from build123d import *

# Parameters (mm, degrees)
ESQUISSE1_R          = 1.65
ESQUISSE1_R_2        = 3.5
SHAPE_DEPTH          = 10
ESQUISSE6_W          = 10
ESQUISSE6_H          = 15
MAINSHAPE_DEPTH      = 30.25
ESQUISSE10_W         = 13.5
ESQUISSE10_H         = 12.85118471
SPACEREMOVER_DEPTH   = 13
ESQUISSE11_R         = 2.25
AXE_DEPTH            = 16
ESQUISSE12_R         = 3.7
BEARINGBOTTOM_DEPTH  = 3.2
BEARINGTOP_START     = -3.4
ESQUISSE14_R         = 3.7
BEARINGTOP_DEPTH     = 3.4
ESQUISSE15_R         = 2.25
AXEEND_DEPTH         = 1
ESQUISSE16_W         = 3
ESQUISSE16_H         = 7
AXELOCKER_DEPTH      = 10
ESQUISSE17_W         = 30.25
ESQUISSE17_H         = 0.85118471
RENFORCMENT_DEPTH    = 10
ESQUISSE18_W         = 30.25
ESQUISSE18_H         = 2
MASSREMOVER_DEPTH    = 10
CONG_1_R             = 4
ESQUISSE19_R         = 1
REMOVER_HELPER_DEPTH = 10


with BuildPart() as part:
    # Esquisse1 → Shape (new body)
    with BuildSketch(Plane.XY):
        with BuildLine():
            ThreePointArc((5, 10), (0, 15), (-5, 10))
            Line((-5, 10), (-5, -10))
            ThreePointArc((-5, -10), (0, -15), (5, -10))
            Line((5, -10), (5, 10))
        make_face()
        with Locations((0, 10)):
            Circle(ESQUISSE1_R, mode=Mode.SUBTRACT)
        Circle(ESQUISSE1_R_2, mode=Mode.SUBTRACT)
        with Locations((0, -10)):
            Circle(ESQUISSE1_R, mode=Mode.SUBTRACT)
    extrude(amount=SHAPE_DEPTH)

    # Esquisse6 → MainShape (add)
    with BuildSketch(Plane(origin=(5, 0, 0), x_dir=(0, 0, -1), z_dir=(1, 0, 0))):
        with Locations((-5, 0)):
            Rectangle(ESQUISSE6_W, ESQUISSE6_H)
    extrude(amount=MAINSHAPE_DEPTH)

    # Esquisse10 → SpaceRemover (cut)
    with BuildSketch(Plane(origin=(0, 0, 0), x_dir=(-1, 0, 0), z_dir=(0, 0, -1))):
        with Locations((-15.5, 1.074407645)):
            Rectangle(ESQUISSE10_W, ESQUISSE10_H)
    extrude(amount=-SPACEREMOVER_DEPTH, mode=Mode.SUBTRACT)

    # Esquisse11 → Axe (cut)
    with BuildSketch(Plane(origin=(35.25, 0, 0), x_dir=(0, 0, -1), z_dir=(1, 0, 0))):
        with Locations((-5, 0)):
            Circle(ESQUISSE11_R)
    extrude(amount=-AXE_DEPTH, mode=Mode.SUBTRACT)

    # Esquisse12 → BearingBottom (cut)
    with BuildSketch(Plane(origin=(8.75, 0, 0), x_dir=(0, 0, -1), z_dir=(1, 0, 0))):
        with Locations((-5, 0)):
            Circle(ESQUISSE12_R)
    extrude(amount=-BEARINGBOTTOM_DEPTH, mode=Mode.SUBTRACT)

    # Esquisse14 → BearingTop (cut)
    with BuildSketch(Plane.ZY.offset(-22.25).offset(BEARINGTOP_START)):
        with Locations(Location((5, 0, 0), (0, 0, 180))):
            Circle(ESQUISSE14_R)
    extrude(amount=BEARINGTOP_DEPTH, mode=Mode.SUBTRACT)

    # Esquisse15 → AxeEnd (cut)
    with BuildSketch(Plane(origin=(5.55, 0, 0), x_dir=(0, 0, -1), z_dir=(1, 0, 0))):
        with Locations((-5, 0)):
            Circle(ESQUISSE15_R)
    extrude(amount=-AXEEND_DEPTH, mode=Mode.SUBTRACT)

    # Esquisse16 → AxeLocker (cut)
    with BuildSketch(Plane(origin=(0, 0, 0), x_dir=(-1, 0, 0), z_dir=(0, 0, -1))):
        with Locations((-30.45, 0)):
            Rectangle(ESQUISSE16_W, ESQUISSE16_H)
    extrude(amount=-AXELOCKER_DEPTH, mode=Mode.SUBTRACT)

    # Esquisse17 → Renforcment (add)
    with BuildSketch(Plane(origin=(0, 0, 0), x_dir=(-1, 0, 0), z_dir=(0, 0, -1))):
        with Locations((-20.125, -7.925592355)):
            Rectangle(ESQUISSE17_W, ESQUISSE17_H)
    extrude(amount=-RENFORCMENT_DEPTH)

    # Esquisse18 → MassRemover (cut)
    with BuildSketch(Plane(origin=(0, 0, 0), x_dir=(-1, 0, 0), z_dir=(0, 0, -1))):
        with Locations((-20.125, 6.5)):
            Rectangle(ESQUISSE18_W, ESQUISSE18_H)
    extrude(amount=-MASSREMOVER_DEPTH, mode=Mode.SUBTRACT)

    # Congé1
    cong_1_edges = [part.edges().sort_by_distance(p)[0] for p in [
        (35.25, -8.35118471, 5),
        (5, -8.35118471, 5),
    ]]
    fillet(cong_1_edges, radius=CONG_1_R)

    # Esquisse19 → Remover helper (cut)
    with BuildSketch(Plane(origin=(4.55, 0, 0), x_dir=(0, 0, -1), z_dir=(1, 0, 0))):
        with Locations((-5, 0)):
            Circle(ESQUISSE19_R)
    extrude(amount=-REMOVER_HELPER_DEPTH, mode=Mode.SUBTRACT)


solid = part.part
Geometry: final body of the model. Coordinates: model frame, mm. A direction names the side the tool comes from. Give positions to 0.01 mm unless a question says otherwise; leave off trailing zeros. Order: outer loops, then holes, each group sorted by start corner. A loop starts at its lowest first (then second) coordinate and runs counter-clockwise, first axis right, second up. Notation, with made-up numbers: (56.5, -1.5) - (66.5, -1.5) arc R22 ccw to (66.5, 33.5) - close; hole circle Ø3 at (44.5, 54). An arc over 180 degrees is marked (long way). Use CSV: the item, a comma, the result in double quotes.
1. Section query A-A (x = 0). Output: boundary loops of the cut face in (y, z), plus the area to 3 significant figures.
Answers below:
outline,"(-15, 0) - (-11.65, 0) - (-11.65, 10) - (-15, 10) - close; (-8.35, 0) - (-3.5, 0) - (-3.5, 10) - (-8.35, 10) - close; (3.5, 0) - (8.35, 0) - (8.35, 10) - (3.5, 10) - close; (11.65, 0) - (15, 0) - (15, 10) - (11.65, 10) - close"
area,"164 mm2"
2. Access query for faces 5 (the face through (16, -5.351, 5)), 6 (the face through (23.97, -1.11, 1.47)), 7 (the face through (7, 5.5, 5)). Directions: +Z, -Z, +X, -X, +Y, -Y. A direction counts if a zero-diameter tool reaches every point of the face in a straight line with its end or side. Return the directions, or none.
Answers below:
face 5,"+Z, -Z, +Y"
face 6,"none"
face 7,"+Z, -Z, +X, +Y"
3. Section query C-C (z = 5). Give the number of separate pieces and of enclosed holes in the cut face, plus the area to 3 significant figures.
Answers below:
separate pieces,"3"
enclosed holes,"2"
area,"385 mm2"
4. Contact query for flat-ended pins moving along their axis: pin 1 (4 mm diameter, centred on x = 0, y = 10, fed in from -Z); pin 2 (4 mm diameter, centred on x = 0, y = 0, fed in from -Z); pin 3 (1 mm diameter, centred on x = 17.5, z = 3.5, fed in from +Y); pin 4 (2.5 mm diameter, centred on x = 30.5, z = 3.5, fed in from -Y). Output: stop coordinate, or through.
Answers below:
pin 1,"z = 0"
pin 2,"through"
pin 3,"y = -5.35"
pin 4,"y = -8.35"
5. Section query D-D (x = 26.5). Output: boundary loops of the cut face in (y, z).
Answers below:
outline,"(-8.35, 0) - (5.5, 0) - (5.5, 10) - (-8.35, 10) - close; hole circle Ø4.5 at (0, 5)"
6. Section query B-B (y = 5). Output: boundary loops of the cut face in (x, z), plus the area to 4 significant figures.
Answers below:
outline,"(-5, 0) - (8.75, 0) - (8.75, 10) - (-5, 10) - close; (22.25, 0) - (35.25, 0) - (35.25, 10) - (22.25, 10) - close"
area,"267.5 mm2"
7. Mould query, pull axis Y, two halves, no side actions, for faces 1 (the face through (8.75, 4, 4)), 2 (the face through (7.172, -1.417, 1.582)), 3 (the face through (4.55, 1, 4)), 4 (the face through (20, -8.351, 5)). Classes: +Y half, -Y half, draft (parallel to the pull), parting line (faces both ways), or undercut.
Answers below:
face 1,"draft"
face 2,"undercut"
face 3,"undercut"
face 4,"-Y half"
8. Material intervals for line 1 along X through (y, z) = (-1, 8.75); line 2 along Y through (x, z) = (26.5, 5); line 3 along X through (y, z) = (5, 7.5), sorted ascending. Write a range as from..to.
Answers below:
line 1,"-5..-3.35, 3.35..8.75, 22.25..28.95, 31.95..35.25"
line 2,"-8.35..-2.25, 2.25..5.5"
line 3,"-5..8.75, 22.25..35.25"
